Check sheet for the modelled part. Datum: model origin and axes. Units: mm. Face numbers are marked on the shaded views. A direction names the side the tool comes from. Round coordinates to 2 decimals unless told otherwise and drop trailing zeros. Write each loop counter-clockwise with the first axis right and the second up, starting at its lowest first coordinate (ties: lowest second). Pieces come first, ordered by that corner, then holes.
Item 1: Depth check by flat-ended pin: pin 1 (5 mm diameter, centred on y = 8.5, z = -8, fed in from -X); pin 2 (5 mm diameter, centred on x = 4.5, z = 8, fed in from +Y). Enter the tip coordinate at first touch or a pass-through.
Item 2: Section check A-A, the plane y = 5.5. Record the cut outline in (x, z), plus the area to 3 significant figures.
Item 3: Section check B-B, the plane z = 8. Record the cut outline in (x, y), plus the area to 3 significant figures.
Item 4: Release check for a two-part mould opening along Z. For the marked faces 3, 4 and 5 record: pulls with the +Z half, pulls with the -Z half, needs draft (parallel to the pull), parting line crosses it, or undercut.
Item 5: Material ranges on line 1 along Z through (x, y) = (4.5, 1); line 2 along X through (y, z) = (3.75, -0.25); line 3 along Y through (x, z) = (23.5, 10), recorded low to high.
Item 6: Section check C-C, the plane x = 4.5. Record the cut outline in (y, z).
Item 7: Section check D-D, the plane y = 3.5. Record the cut outline in (x, z).
Item 8: Set-up check for the marked faces 1 and 2: record each of +Z, -Z, +X, -X, +Y, -Y from which the full face is reachable in a straight line by a thin tool's end or side.
from build123d import *

# Parameters (mm, degrees)
F0_W     = 3
F0_H     = 7
F1_DEPTH = 12.5
F2_R     = 1.5
F3_DEPTH = 25.4
F4_R     = 1.5
F5_DEPTH = 25.4


with BuildPart() as f1:
    # F0 (on Top) → F1 (new body, symmetric)
    with BuildSketch(Plane.XY):
        Polygon((0, 3), (0, 0), (41, 0), (41, 3), (38, 3), align=None)
        with Locations((39.5, 6.5)):
            Rectangle(F0_W, F0_H)
    extrude(amount=F1_DEPTH, both=True)

    # F2 (on face) → F3 (cut)
    with BuildSketch(Plane.XZ):
        with Locations((4.5, 8)):
            Circle(F2_R)
        with Locations((4.5, -8)):
            Circle(F2_R)
    extrude(amount=-F3_DEPTH, mode=Mode.SUBTRACT)

    # F4 (on face) → F5 (cut)
    with BuildSketch(Plane.YZ.offset(41)):
        with Locations((5.5, 8)):
            Circle(F4_R)
        with Locations((5.5, -8)):
            Circle(F4_R)
    extrude(amount=-F5_DEPTH, mode=Mode.SUBTRACT)


solid = f1.part
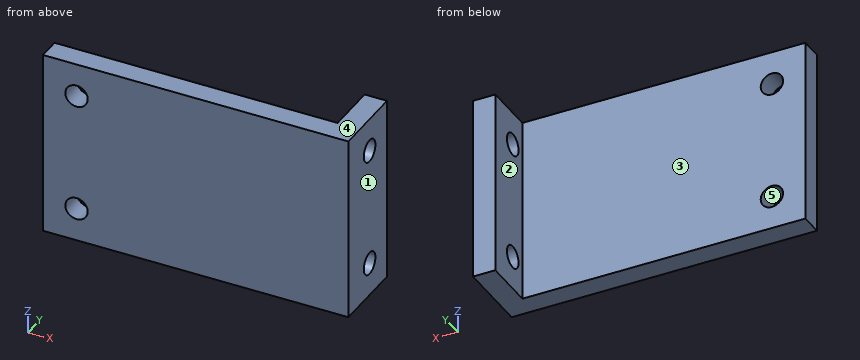
Values found:
1. pin 1: stops at x = 38
1. pin 2: stops at y = 3
2. outline: (38, -12.5) - (41, -12.5) - (41, -9.5) - (38, -9.5) - close; (38, -6.5) - (41, -6.5) - (41, 6.5) - (38, 6.5) - close; (38, 9.5) - (41, 9.5) - (41, 12.5) - (38, 12.5) - close
2. area: 57.0 mm2
3. outline: (0, 0) - (3, 0) - (3, 3) - (0, 3) - close; (6, 0) - (41, 0) - (41, 4) - (38, 4) - (38, 3) - (6, 3) - close; (38, 7) - (41, 7) - (41, 10) - (38, 10) - close
3. area: 126 mm2
4. face 3: needs draft
4. face 4: pulls with the +Z half
4. face 5: undercut
5. line 1: z = -12.5 to -9.5, -6.5 to 6.5, 9.5 to 12.5
5. line 2: x = 38 to 41
5. line 3: y = 0 to 3
6. outline: (0, -12.5) - (3, -12.5) - (3, -9.5) - (0, -9.5) - close; (0, -6.5) - (3, -6.5) - (3, 6.5) - (0, 6.5) - close; (0, 9.5) - (3, 9.5) - (3, 12.5) - (0, 12.5) - close
7. outline: (38, -12.5) - (41, -12.5) - (41, 12.5) - (38, 12.5) - close
8. face 1: +Z, -Z, +X, +Y, -Y
8. face 2: +Z, -Z, -X, +Y
